Check sheet for the modelled part. Datum: model origin and axes. Units: mm. Face numbers are marked on the shaded views. Round coordinates to 2 decimals unless told otherwise and drop trailing zeros. Write each loop counter-clockwise with the first axis right and the second up, starting at its lowest first coordinate (ties: lowest second). Pieces come first, ordered by that corner, then holes.
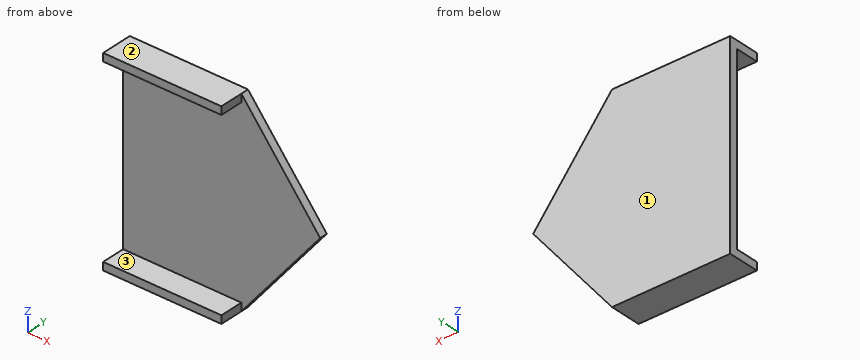
from build123d import *

# Parameters (mm, degrees)
BOSS_EXTRUDE1_DEPTH = 5
SKETCH2_W           = 150
SKETCH2_H           = 30
BOSS_EXTRUDE2_DEPTH = 10


with BuildPart() as part:
    # Sketch1 → Boss-Extrude1 (new, symmetric)
    with BuildSketch(Plane(origin=(0, 0, 0), x_dir=(1, 0, 0), z_dir=(0, 1, 0))):
        Polygon((75, 125), (175, 0), (75, -125), (-75, -125), (-75, 125), align=None)
    extrude(amount=BOSS_EXTRUDE1_DEPTH, both=True)

    # Sketch2 → Boss-Extrude2 (add)
    with BuildSketch(Plane(origin=(0, 0, -125), x_dir=(-1, 0, 0), z_dir=(0, 0, -1))):
        with Locations((0, -20)):
            Rectangle(SKETCH2_W, SKETCH2_H)
    boss_extrude2 = extrude(amount=-BOSS_EXTRUDE2_DEPTH)

    # Mirror1: Boss-Extrude2 across plane
    add(boss_extrude2.mirror(Plane.XY))


solid = part.part
1. Go/stop test with flat-tipped pins: pin 1 (2 mm diameter, centred on x = 94, y = -4, fed in from +Z); pin 2 (8 mm diameter, centred on y = -15, z = -119, fed in from +X); pin 3 (12 mm diameter, centred on x = 23.5, z = 14.5, fed in from -Y); pin 4 (1 mm diameter, centred on y = -7, z = -38, fed in from -X). Record where each tip stops, or that it passes through.
2. Sectioned sample at A-A, the plane y = -21.5. Enter the section's corners in (x, z), plus the area to 3 significant figures.
3. Sectioned sample at D-D, the plane z = 108. Enter the section's corners in (x, y), plus the area to 3 significant figures.
4. Scan lines: line 1 along Z through (x, y) = (24.5, -12); line 2 along Y through (x, z) = (-55.5, 36); line 3 along X through (y, z) = (-2.5, 93). Record each from-to range of solid material in increasing order.
5. Sectioned sample at C-C, the plane x = 3.5. Enter the section's corners in (y, z).
6. Release check for a two-part mould opening along Z. For the marked faces 1, 2 and 3 record: released by +Z, released by -Z, zero draft, split by the parting line, or undercut.
7. Sectioned sample at B-B, the plane y = 0. Enter the section's corners in (x, z), plus the area to 3 significant figures.
Computed values:
1. pin 1: stops at z = 102.5
1. pin 2: stops at x = 75
1. pin 3: stops at y = -5
1. pin 4: passes through
2. outline: (-75, -125) - (75, -125) - (75, -115) - (-75, -115) - close; (-75, 115) - (75, 115) - (75, 125) - (-75, 125) - close
2. area: 3,000 mm2
3. outline: (-75, -5) - (88.6, -5) - (88.6, 5) - (-75, 5) - close
3. area: 1,640 mm2
4. line 1: z = -125 to -115, 115 to 125
4. line 2: y = -5 to 5
4. line 3: x = -75 to 100.6
5. outline: (-35, -125) - (5, -125) - (5, 125) - (-35, 125) - (-35, 115) - (-5, 115) - (-5, -115) - (-35, -115) - close
6. face 1: zero draft
6. face 2: released by +Z
6. face 3: undercut
7. outline: (-75, -125) - (75, -125) - (175, 0) - (75, 125) - (-75, 125) - close
7. area: 50,000 mm2
